```python
from build123d import *

# Parameters (mm, degrees)
SKETCH_1_W      = 30
SKETCH_1_H      = 37
SKETCH_1_R      = 1.05
SKETCH_1_R_2    = 0.45
EXTRUDE_1_DEPTH = 1.6
SKETCH_2_W      = 12.1
SKETCH_2_H      = 9.4
EXTRUDE_2_DEPTH = 1
SKETCH_3_W      = 15.5
SKETCH_3_H      = 5.1
EXTRUDE_3_DEPTH = 2


with BuildPart() as part:
    # 草图1 → 凸台-拉伸1 (new body)
    with BuildSketch(Plane(origin=(0, 0, 0), x_dir=(1, 0, 0), z_dir=(0, 1, 0))):
        with Locations((15, -18.5)):
            Rectangle(SKETCH_1_W, SKETCH_1_H)
        with Locations(Location((2, -2, 0), (0, 0, 270))):
            Circle(SKETCH_1_R, mode=Mode.SUBTRACT)
        with Locations(Location((28, -2, 0), (0, 0, 270))):
            Circle(SKETCH_1_R, mode=Mode.SUBTRACT)
        with Locations(Location((2, -35, 0), (0, 0, 270))):
            Circle(SKETCH_1_R, mode=Mode.SUBTRACT)
        with Locations(Location((28, -35, 0), (0, 0, 270))):
            Circle(SKETCH_1_R, mode=Mode.SUBTRACT)
        with Locations(Location((7, -10.5, 0), (0, 0, 270))):
            Circle(SKETCH_1_R_2, mode=Mode.SUBTRACT)
        with Locations(Location((23, -10.5, 0), (0, 0, 270))):
            Circle(SKETCH_1_R_2, mode=Mode.SUBTRACT)
        with Locations(Location((7, -26.5, 0), (0, 0, 270))):
            Circle(SKETCH_1_R_2, mode=Mode.SUBTRACT)
        with Locations(Location((23, -26.5, 0), (0, 0, 270))):
            Circle(SKETCH_1_R_2, mode=Mode.SUBTRACT)
        with Locations(Location((5, -18.5, 0), (0, 0, 270))):
            Circle(SKETCH_1_R, mode=Mode.SUBTRACT)
        with Locations(Location((25, -18.5, 0), (0, 0, 270))):
            Circle(SKETCH_1_R, mode=Mode.SUBTRACT)
    extrude(amount=EXTRUDE_1_DEPTH)

    # 草图2 → 凸台-拉伸2 (add)
    with BuildSketch(Plane(origin=(0, 1.6, 0), x_dir=(1, 0, 0), z_dir=(0, 1, 0))):
        with Locations((14.85, -18.7)):
            Rectangle(SKETCH_2_W, SKETCH_2_H)
    extrude(amount=EXTRUDE_2_DEPTH)

    # 草图3 → 凸台-拉伸3 (add)
    with BuildSketch(Plane(origin=(0, 1.6, 0), x_dir=(1, 0, 0), z_dir=(0, 1, 0))):
        with Locations((14.95, -3.85)):
            Rectangle(SKETCH_3_W, SKETCH_3_H)
    extrude(amount=EXTRUDE_3_DEPTH)


solid = part.part
```
Model file for the job. Use its own axes, mm. A direction names the side the tool comes from. Round coordinates to 2 decimals unless told otherwise and drop trailing zeros. Write each loop counter-clockwise with the first axis right and the second up, starting at its lowest first coordinate (ties: lowest second). Pieces come first, ordered by that corner, then holes. Notation, with made-up numbers: M 31,-40 L 68,-40 A22 ccw 68,-5 Z; hole C 33,3 d5. An arc over 180 degrees is marked long. Put each result on its own line as item: value.
Item 1: Cut at C-C (y = 0.7). State how many separate pieces and enclosed holes the cut face has, and give its area (3 significant figures).
Responses:
separate pieces: 1
enclosed holes: 10
area: 1,090 mm²
Item 2: Probe L1, parallel to X at y = 1, z = 2; L2, parallel to X at y = 0.45, z = 26.5; L3, parallel to Z at x = 23, y = 1.2. List the from-to ranges inside material, lowest first. Write a range as from..to.
Responses:
L1: 0..0.95, 3.05..26.95, 29.05..30
L2: 0..6.55, 7.45..22.55, 23.45..30
L3: 0..10.05, 10.95..26.05, 26.95..37
Item 3: Flat gauge pins, fed straight in: P1, Ø4.5, axis at x = 13, z = 17.5, coming from the +Y side; P2, Ø1.1, axis at x = 14, y = 2.5, coming from the +Z side; P3, Ø1.6, axis at y = 2.5, z = 2.5, coming from the -X side; P4, Ø1.9, axis at x = 2, z = 35, coming from the -Y side (3 decimals). Where does each tip first touch, or does it go through?
Responses:
P1: y = 2.6
P2: z = 23.4
P3: x = 7.2
P4: through
Item 4: Tool access for faces 4 (the flat face through (15, 3, 1.3)), 5 (the flat face through (15, 3, 6.4)), 6 (the flat face through (7.2, 3, 4)), 7 (the flat face through (15, 2.6, 19)): list every direction of +Z, -Z, +X, -X, +Y, -Y with a clear straight run to the whole face (end or side of a thin tool).
Responses:
face 4: -Z, +X, -X, +Y
face 5: +X, -X, +Y
face 6: +Z, -Z, -X, +Y
face 7: +Z, +X, -X, +Y
Item 5: Mould opens along Z. For faces 1 (the flat face through (15, 1, 37)), 2 (the cylindrical face through (26.975, 0.789, 1.772)), 3 (the flat face through (15, 1, 0)) say: +Z half, -Z half, draft (parallel to the pull), parting line (faces both ways), or undercut.
Responses:
face 1: +Z half
face 2: undercut
face 3: -Z half
Item 6: Cut at A-A (x = 2). List the corners of the cut face in (y, z).
Responses:
outline: M 0,0 L 1.6,0 L 1.6,0.95 L 0,0.95 Z; M 0,3.05 L 1.6,3.05 L 1.6,33.95 L 0,33.95 Z; M 0,36.05 L 1.6,36.05 L 1.6,37 L 0,37 Z
Item 7: Cut at D-D (x = 25). List the corners of the cut face in (y, z), and give its area (3 significant figures).
Responses:
outline: M 0,0 L 1.6,0 L 1.6,17.45 L 0,17.45 Z; M 0,19.55 L 1.6,19.55 L 1.6,37 L 0,37 Z
area: 55.8 mm²
Item 8: Cut at B-B (z = 18.5). List the corners of the cut face in (x, y), and give its area (3 significant figures).
Responses:
outline: M 0,0 L 3.95,0 L 3.95,1.6 L 0,1.6 Z; M 6.05,0 L 23.95,0 L 23.95,1.6 L 20.9,1.6 L 20.9,2.6 L 8.8,2.6 L 8.8,1.6 L 6.05,1.6 Z; M 26.05,0 L 30,0 L 30,1.6 L 26.05,1.6 Z
area: 53.4 mm²
